Autodesk Inventor part; units mm, degrees
ref_plane "YZ Plane" through (0, 0, 0) normal (1, 0, 0) x (0, 1, 0)
ref_plane "XZ Plane" through (0, 0, 0) normal (0, 1, 0) x (-1, 0, 0)
ref_plane "XY Plane" through (0, 0, 0) normal (0, 0, 1) x (1, 0, 0)
sketch "Sketch1" plane through (0, 0, 0) normal (0, 0, 1) x (1, 0, 0)
  line L0 (0, 0) -> (0, 35)
  line L1 (0, 35) -> (5, 35)
  line L2 (5, 35) -> (5, 5)
  line L3 (5, 5) -> (73, 5)
  line L4 (73, 5) -> (73, 35)
  line L5 (73, 35) -> (78, 35)
  line L6 (78, 35) -> (78, 0)
  line L7 (78, 0) -> (0, 0)
  dimension "d0" = 35
  dimension "d1" = 5
  dimension "d2" = 30
  dimension "d3" = 68
  dimension "d4" = 5
extrude "Extrusion1" add sketch "Sketch1" along normal blind 30
sketch "Sketch2" plane through (5, 5, 0) normal (1, 0, 0) x (0, 0, -1)
  circle A0 centre (-15, 17.5) radius 5
  line L0 (0, -5) -> (0, 30)
  line L1 (0, 30) -> (-30, 30)
  dimension "d7" = 10
  dimension "d8" = 15
  dimension "d9" = 12.5
extrude "Extrusion2" cut sketch "Sketch2" along normal mid plane 1000
sketch "Sketch3" plane through (5, 5, 0) normal (0, 1, 0) x (1, 0, 0)
  circle A0 centre (8, -15) radius 3.625
  line L0 (68, 0) -> (0, 0)
  line L1 (0, 0) -> (0, -30)
  circle A1 centre (60, -15) radius 3.625
  line L2 (68, 0) -> (68, -30)
  point P0 (-5, 0)
  dimension "d12" = 7.25
  dimension "d13" = 15
  dimension "d14" = 8
  dimension "d15" = 7.25
  dimension "d16" = 8
  dimension "d17" = 15
extrude "Extrusion3" cut sketch "Sketch3" against normal blind 2.1735 draft -45
sketch "Sketch4" plane through (13, 2.8265, 15) normal (0, 1, 0) x (1, 0, 0)
  circle A0 centre (0, 0) radius 1.4515
  circle A1 centre (0, 0) radius 1.4515
  circle A2 centre (52, 0) radius 1.4515
  circle A3 centre (52, 0) radius 1.4515
  point P0 (-13, 15)
extrude "Extrusion4" cut sketch "Sketch4" against normal blind 10
sketch "Sketch5" plane through (5, 5, 0) normal (0, 1, 0) x (1, 0, 0)
  line L0 (20, -7.5) -> (48, -7.5)
  line L1 (48, -7.5) -> (48, -22.5)
  line L2 (48, -22.5) -> (20, -22.5)
  line L3 (20, -22.5) -> (20, -7.5)
  line L4 (20, -7.5) -> (48, -22.5) construction
  line L5 (48, -7.5) -> (20, -22.5) construction
  line L6 (68, 0) -> (0, 0)
  line L7 (0, 0) -> (0, -30)
  point P0 (-5, 0)
  point P1 (34, -15)
  dimension "d22" = 28
  dimension "d23" = 15
  dimension "d24" = 15
  dimension "d25" = 34
extrude "Extrusion5" cut sketch "Sketch5" against normal through all
properties part number "1st arm to next clamp"
Could you check a few things on this model? Use its own coordinates, in mm. A direction names the side the tool comes from. Give positions to 0.01 mm unless a question says otherwise; leave off trailing zeros. Order: outer loops, then holes, each group sorted by start corner. A loop starts at its lowest first (then second) coordinate and runs counter-clockwise, first axis right, second up.
Q1. If I drill on line 1 along X through (y, z) = (30.5, 27); line 2 along Y through (x, z) = (3.05, 15); line 3 along X through (y, z) = (1.2, 15), over which ranges is the centre line in solid material (lowest first)?
Q2. Suppose I cut it at A-A, the plane y = 10. Write out the boundary of the cut face in (x, z).
Q3. For faces 4 (the flat face through (73, 16, 15)), 5 (the flat face through (39, 3, 22.5)), 6 (the flat face through (2, 35, 15)), which set-ups out of +Z, -Z, +X, -X, +Y, -Y let a thin tool reach every point of the face, with its end or its side?
Q4. We'd pull the mould along Y, two halves only. Please class faces 1 (the flat face through (75, 35, 15)), 2 (the cylindrical face through (75.46, 27.38, 16.08)), 3 (the flat face through (53, 3, 15)): +Y half, -Y half, draft (parallel to the pull), parting line (faces both ways), or undercut.
Q5. I'm going to push a flat-ended pin straight in: P1, Ø10, axis at x = 12, z = 14.5, coming from the +Y side. Where does the tip first touch, or does it pass through?
Q6. Suppose I cut it at C-C, the plane x = 31. Write out the boundary of the cut face in (y, z), and give its area (3 significant figures).
Q7. Suppose I cut it at D-D, the plane y = 22.5. Write out the boundary of the cut face in (x, z).
Q8. Suppose I cut it at B-B, the plane z = 15. Count the separate pieces of the cut face and the enclosed holes in it, and give its area (3 significant figures).
Solution:
1. line 1: x = 0 to 5, 73 to 78
1. line 2: y = 0 to 17.5, 27.5 to 35
1. line 3: x = 0 to 11.55, 14.45 to 25, 53 to 63.55, 66.45 to 78
2. outline: (0, 0) - (5, 0) - (5, 30) - (0, 30) - close; (73, 0) - (78, 0) - (78, 30) - (73, 30) - close
3. face 4: +Z, -Z, +Y
3. face 5: +Y, -Y
3. face 6: +Z, -Z, +X, -X, +Y
4. face 1: +Y half
4. face 2: undercut
4. face 3: draft
5. P1: stops at y = 5
6. outline: (0, 0) - (5, 0) - (5, 7.5) - (0, 7.5) - close; (0, 22.5) - (5, 22.5) - (5, 30) - (0, 30) - close
6. area: 75.0 mm2
7. outline: (0, 0) - (5, 0) - (5, 10) - (0, 10) - close; (0, 20) - (5, 20) - (5, 30) - (0, 30) - close; (73, 0) - (78, 0) - (78, 10) - (73, 10) - close; (73, 20) - (78, 20) - (78, 30) - (73, 30) - close
8. separate pieces: 6
8. enclosed holes: 0
8. area: 412 mm2
